Answer from the drawing. Dimensions are ordinates in mm from the lowest x, y and z of the part. A direction names the side the tool comes from. Give positions to 0.01 mm unless a question says otherwise; leave off trailing zeros. Order: outer loops, then holes, each group sorted by start corner. A loop starts at its lowest first (then second) coordinate and runs counter-clockwise, first axis right, second up. Notation, with made-up numbers: (70, 64.5) - (112, 64.5) arc R21 cw to (112, 94.5) - close; hole circle Ø9 at (22, 67). An arc over 180 degrees is marked (long way). Answer in a Markdown table with one row per item.
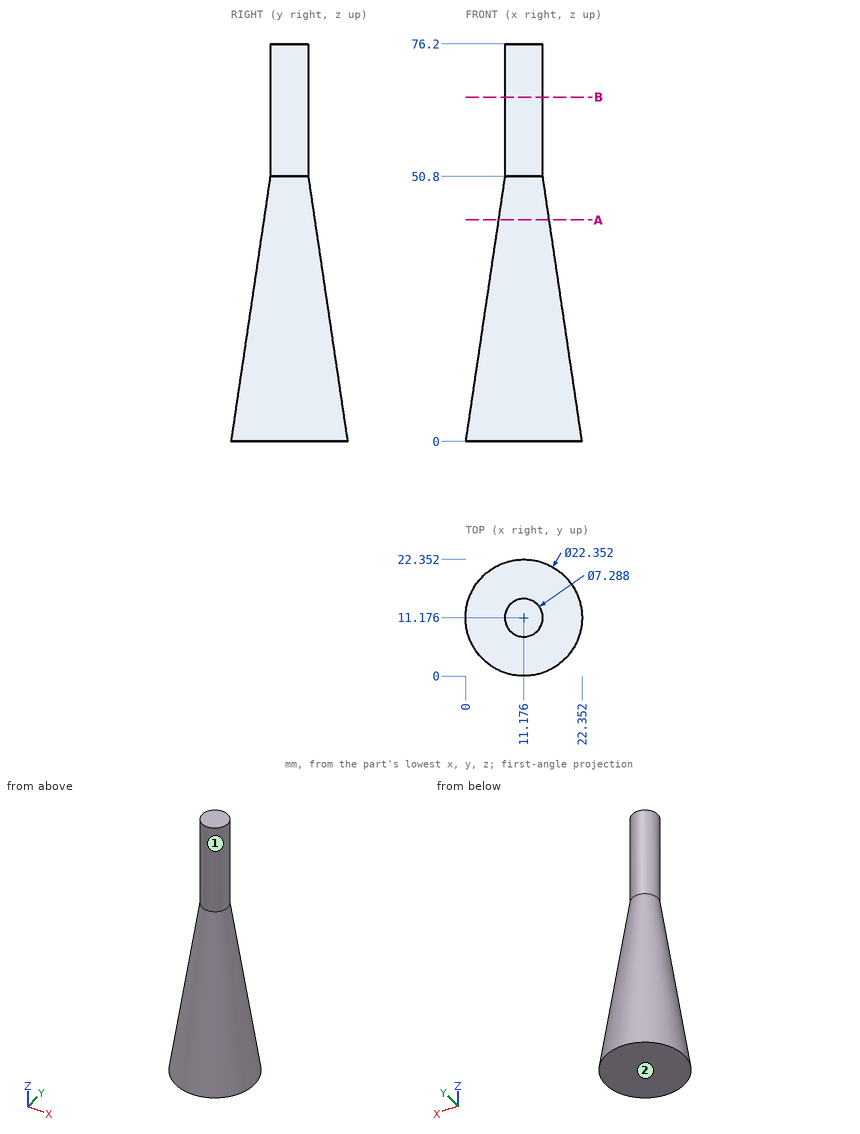
Item 1: Consider line 1 (X direction, y = 11.5, z = 55) (1 decimal); line 2 (Y direction, x = 7.5, z = 31.5); line 3 (X direction, y = 7, z = 42.5). Determine where each line is inside the solid, lowest interval first.
Answer block:
| item | result |
|---|---|
| line 1 | 7.5 to 14.8 |
| line 2 | 5.81 to 16.54 |
| line 3 | 8.66 to 13.69 |
Item 2: Find section B-B on z = 66. Write down the section's boundary in (x, y).
Answer block:
| item | result |
|---|---|
| outline | circle Ø7.29 at (11.18, 11.18) |
Item 3: Find section A-A on z = 42.5. Write down the section's boundary in (x, y) (1 decimal).
Answer block:
| item | result |
|---|---|
| outline | circle Ø9.7 at (11.2, 11.2) |
Item 4: Each of these flat-tipped pins is pushed along its axis until it touches: P1, Ø1, axis at x = 12, z = 18, coming from the +Y side; P2, Ø6, axis at x = 13, z = 62.5, coming from the +Y side; P3, Ø4, axis at y = 5.5, z = 25.5, coming from the +X side. Where does it stop, or does it pass through?
Answer block:
| item | result |
|---|---|
| P1 | y = 19.73 |
| P2 | y = 14.82 |
| P3 | x = 17.64 |
Item 5: Which of the six approach directions +Z, -Z, +X, -X, +Y, -Y give full straight-line access (tool end or side, diameter ignored) to the marked faces 1 and 2?
Answer block:
| item | result |
|---|---|
| face 1 | +Z |
| face 2 | -Z, +X, -X, +Y, -Y |
